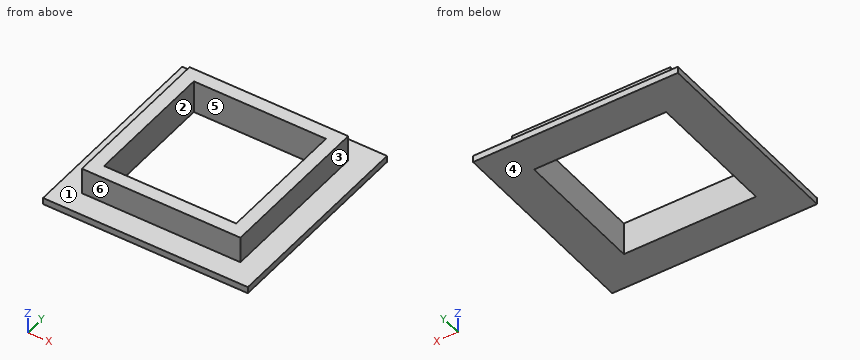
from build123d import *

# Parameters (mm, degrees)
F0_W     = 9.6
F0_H     = 9.6
F1_DEPTH = 2
F2_T     = -0.8
F0_W_2   = 12.4
F0_H_2   = 12.4
F3_DEPTH = 0.4
F4_DEPTH = 1


with BuildPart() as f1:
    # F0 (on Top) → F1 (new body)
    with BuildSketch(Plane.XY):
        Rectangle(F0_W, F0_H)
    extrude(amount=F1_DEPTH)

    # F2
    f2_openings = [f1.faces().sort_by_distance(p)[0] for p in [
        (0, 0, 2),
    ]]
    offset(amount=F2_T, openings=f2_openings)

    # F0 (on Top) → F3 (join)
    with BuildSketch(Plane.XY):
        Rectangle(F0_W_2, F0_H_2)
        Rectangle(F0_W, F0_H, mode=Mode.SUBTRACT)
    extrude(amount=F3_DEPTH)

    # F4 (cut): a face of the model
    f4_faces = [f1.faces().sort_by_distance(p)[0] for p in [
        (0, 0, 0.8),
    ]]
    extrude(f4_faces, amount=-F4_DEPTH, mode=Mode.SUBTRACT)


solid = f1.part
Work out the finished part from the listing and answer in its coordinate system (mm). Face numbers are marked on the shaded views. A direction names the side the tool comes from. Coordinates: 2 decimals unless noted, no trailing zeros. Order: outer loops, then holes, each group sorted by start corner. A loop starts at its lowest first (then second) coordinate and runs counter-clockwise, first axis right, second up. Notation, with made-up numbers: (41.5, 20) - (58.5, 20) arc R34 ccw to (58.5, 54) - close; hole circle Ø9 at (-4.75, -1.5). An arc over 180 degrees is marked (long way). Put each result on its own line as item: value. Start each with the question number.
1) Find section A-A (z = 1.5). Give the vertices of the cut face in (x, y).
2) Find section D-D (x = -4.25). Give the vertices of the cut face in (y, z).
3) Find section B-B (x = -0.75). Give the vertices of the cut face in (y, z).
4) Flat-ended cylindrical pins translate along their axes: pin 1 (0.8 mm diameter, centred on x = -0.5, z = 1.5, fed in from -Y); pin 2 (1 mm diameter, centred on y = -0.5, z = 1, fed in from +X); pin 3 (0.5 mm diameter, centred on x = 2, z = 1.5, fed in from +Y). Find the tip coordinate at first contact, or state that the pin passes through.
5) Find the intervals of material crossed by line 1 (X direction, y = -0.75, z = 0.55); line 2 (Y direction, x = 1, z = 0.2), in increasing order. Write a range as from..to.
6) For a pull along X with two mould halves and no side action, classify the marked faces 1, 2 and 3 as released by +X, released by -X, zero draft, split by the parting line, or undercut.
7) For the marked faces 4, 5 and 6, determine the directions among +Z, -Z, +X, -X, +Y, -Y from which every point of the face is accessible in a straight line to the end or side of a thin tool.
Results list:
1. outline: (-4.8, -4.8) - (4.8, -4.8) - (4.8, 4.8) - (-4.8, 4.8) - close; hole (-4, -4) - (4, -4) - (4, 4) - (-4, 4) - close
2. outline: (-6.2, 0) - (6.2, 0) - (6.2, 0.4) - (4.8, 0.4) - (4.8, 2) - (-4.8, 2) - (-4.8, 0.4) - (-6.2, 0.4) - close
3. outline: (-6.2, 0) - (-4, 0) - (-4, 2) - (-4.8, 2) - (-4.8, 0.4) - (-6.2, 0.4) - close; (4, 0) - (6.2, 0) - (6.2, 0.4) - (4.8, 0.4) - (4.8, 2) - (4, 2) - close
4. pin 1: stops at y = -4.8
4. pin 2: stops at x = 4.8
4. pin 3: stops at y = 4.8
5. line 1: x = -4.8..-4, 4..4.8
5. line 2: y = -6.2..-4, 4..6.2
6. face 1: zero draft
6. face 2: undercut
6. face 3: released by +X
7. face 4: -Z, +X, -X, +Y, -Y
7. face 5: +Z, -Z
7. face 6: +Z, +X, -X, -Y
